```python
from build123d import *

# Parameters (mm, degrees)
BOSS_EXTRUDE1_DEPTH                               = 3.048
BOSS_EXTRUDE2_DEPTH                               = 29.971999999999998
BOSS_EXTRUDE3_DEPTH                               = 3.048
BOSS_EXTRUDE4_DEPTH                               = 3.048
SKETCH13_W                                        = 29.972
SKETCH13_H                                        = 48.7
BOSS_EXTRUDE5_DEPTH                               = 3.048
CSK_FOR_4_FLAT_HEAD_MACHINE_SCREW_100_D           = 2.9464
CSK_FOR_4_FLAT_HEAD_MACHINE_SCREW_100_CSINK_D     = 5.715
CSK_FOR_4_FLAT_HEAD_MACHINE_SCREW_100_CSINK_ANGLE = 100
CUT_EXTRUDE1_DEPTH                                = 1.397
CUT_EXTRUDE1_DEPTH_BACK                           = 1.397
SKETCH15_R                                        = 9.184035329670005
SKETCH15_R_2                                      = 8.124741076595411
SKETCH15_R_3                                      = 8.201451240556812
SKETCH15_R_4                                      = 5.810172256980604
BOSS_EXTRUDE6_DEPTH                               = 3.048
CSK_FOR_4_FLAT_HEAD_MACHINE_SCREW1_AT_2_COUNT     = 2
CSK_FOR_4_FLAT_HEAD_MACHINE_SCREW1_AT_2_PITCH     = 35.474094707842795
CSK_FOR_4_FLAT_HEAD_MACHINE_SCREW1_AT_3_COUNT     = 2
CSK_FOR_4_FLAT_HEAD_MACHINE_SCREW1_AT_3_PITCH     = 43.70753982500484
CSK_FOR_4_FLAT_HEAD_MACHINE_SCREW1_AT_4_COUNT     = 2
CSK_FOR_4_FLAT_HEAD_MACHINE_SCREW1_AT_4_PITCH     = 25.069264350610375
CUT_EXTRUDE2_DEPTH                                = 3.048
FILLET3_R                                         = 3.8099999999999996
FILLET4_R                                         = 1.27
SKETCH21_W                                        = 2.540000000000001
SKETCH21_H                                        = 33.02
CUT_EXTRUDE3_DEPTH                                = 77.47
FILLET5_R                                         = 0.508
FILLET6_R                                         = 0.508
SKETCH22_W                                        = 123.04970813102194
SKETCH22_H                                        = 134.7131875745612
CUT_EXTRUDE4_DEPTH                                = 61.72200000000001


with BuildPart() as part:
    # Sketch2 → Boss-Extrude1 (new body)
    with BuildSketch(Plane.XY):
        Polygon((-47.58059551455695, 48.12489153745831), (-22.21147896413696, 6.554494312375088), (5.701292889255674, 23.58878817682547), (-19.667823661164306, 65.1591854019087), align=None)
        Polygon((-38.85234269167306, 46.0124042215628), (-20.098991648241444, 15.282747135258976), (-3.0269599336282123, 25.701275492720985), (-21.78031097705982, 56.430932579024805), align=None, mode=Mode.SUBTRACT)
    extrude(amount=BOSS_EXTRUDE1_DEPTH)

    # Sketch3 → Boss-Extrude2 (add)
    with BuildSketch(Plane.XY.offset(3.048)):
        Polygon((2.4490708476218597, 21.604058524728963), (-22.920045702798127, 63.17445574981219), (-44.328373472923126, 50.10962118955482), (-18.95925692250314, 8.539223964471608), align=None)
        Polygon((-38.85234269167306, 46.0124042215628), (-20.098991648241444, 15.282747135258976), (-3.0269599336282087, 25.701275492720985), (-21.78031097705982, 56.430932579024805), align=None, mode=Mode.SUBTRACT)
    extrude(amount=BOSS_EXTRUDE2_DEPTH)

    # Sketch4 → Boss-Extrude3 (add)
    with BuildSketch(Plane.XY.offset(33.02)):
        Polygon((-38.85234269167306, 46.0124042215628), (-37.46131723814535, 43.733039051773666), (-20.389285523532113, 54.15156740923567), (-21.78031097705982, 56.430932579024805), align=None)
        Polygon((-29.47566716995725, 30.647575678410885), (-12.403635455344016, 41.0661040358729), (-3.0269599336282087, 25.701275492720985), (-20.098991648241444, 15.282747135258976), align=None)
    extrude(amount=-BOSS_EXTRUDE3_DEPTH)

    # Sketch12 → Boss-Extrude4 (add)
    with BuildSketch(Plane.XY.offset(3.048)):
        Polygon((2.4490708476218597, 21.604058524728963), (5.701292889255674, 23.58878817682547), (8.120429940678708, 25.065112049236276), (-17.248686609741274, 66.6355092743195), (-22.920045702798127, 63.17445574981219), align=None)
    extrude(amount=-BOSS_EXTRUDE4_DEPTH)

    # Sketch13 → Boss-Extrude5 (add)
    with BuildSketch(Plane(origin=(11.391019162328917, 6.95158362794815, 0), x_dir=(0, 0, -1), z_dir=(0.8536015857306615, 0.5209264178731006, 0))):
        with Locations((-18.034000000000002, 41.515472911157566)):
            Rectangle(SKETCH13_W, SKETCH13_H)
    extrude(amount=BOSS_EXTRUDE5_DEPTH)

    # CSK for #4 Flat Head Machine Screw (100)2 (through all)
    with Locations(Plane(origin=(-10.017308607796087, -6.113250932309213, 0), x_dir=(0, 0, 1), z_dir=(-0.8536015857306615, -0.5209264178731007, 0))):
        with Locations((27.397617355, 61.471448289), (7.925915452, 61.471448289), (7.925915452, 21.515515982), (27.397617355, 21.515515982)):
            CounterSinkHole(CSK_FOR_4_FLAT_HEAD_MACHINE_SCREW_100_D / 2, CSK_FOR_4_FLAT_HEAD_MACHINE_SCREW_100_CSINK_D / 2, counter_sink_angle=CSK_FOR_4_FLAT_HEAD_MACHINE_SCREW_100_CSINK_ANGLE)

    # Sketch14 → Cut-Extrude1 (cut, two sides: drawn at the far end of the back side and taken through both)
    with BuildSketch(Plane(origin=(11.607833965104508, 7.083898938087922, 0), x_dir=(0, 0, -1), z_dir=(0.8536015857306615, 0.5209264178731005, 0)).offset(-CUT_EXTRUDE1_DEPTH_BACK)):
        Polygon((-30.697174143874744, 19.61051598216394), (-30.697174143874744, 14.979833054183299), (-24.09806056703731, 14.979833054183299), (-24.09806056703731, 19.610515982163985), (-24.098060567037347, 23.42051598216399), (-27.39761735545604, 25.325515982163957), (-30.697174143874758, 23.420515982163952), align=None)
        Polygon((-27.39761735545604, 57.661448288693826), (-24.098060567037333, 59.56644828869383), (-24.098060567037336, 63.37644828869381), (-24.098060567037336, 70.99644828869384), (-30.69717414387474, 70.99644828869384), (-30.69717414387474, 63.37644828869381), (-30.69717414387474, 59.56644828869381), align=None)
        Polygon((-7.925915451689084, 57.661448288693826), (-4.626358663270381, 59.56644828869382), (-4.626358663270402, 63.37644828869381), (-4.626358663270402, 70.99644828869384), (-11.225472240107786, 70.99644828869384), (-11.225472240107786, 63.376448288693766), (-11.225472240107747, 59.566448288693785), align=None)
        Polygon((-7.925915451689081, 25.325515982163946), (-11.225472240107791, 23.42051598216395), (-11.225472240107791, 19.610515982163946), (-11.225472240107791, 14.979833054183299), (-4.626358663270366, 14.979833054183299), (-4.626358663270366, 19.610515982163953), (-4.6263586632703655, 23.420515982163952), align=None)
    extrude(amount=CUT_EXTRUDE1_DEPTH + CUT_EXTRUDE1_DEPTH_BACK, mode=Mode.SUBTRACT)

    # Sketch15 → Boss-Extrude6 (add)
    with BuildSketch(Plane(origin=(0, 0, 0), x_dir=(-1, 0, 0), z_dir=(0, 0, -1))):
        with Locations((9.758086495919196, 54.36124573948299)):
            Circle(SKETCH15_R)
        with Locations((39.927818301519274, 35.58488100974543)):
            Circle(SKETCH15_R_2)
        with Locations((25.610425726235285, 18.04643091882164)):
            Circle(SKETCH15_R_3)
        with Locations((-3.4576236647063787, 32.70568986323082)):
            Circle(SKETCH15_R_4)
    extrude(amount=-BOSS_EXTRUDE6_DEPTH)

    # Sketch19 → CSK for #4 Flat Head Machine Screw1 (revolve, cut)
    with BuildSketch(Plane(origin=(3.764373982237945, 32.86032278852424, 3.048), x_dir=(0, -1, 0), z_dir=(1, 0, 0))):
        Polygon((0, 0), (-7.5e-16, 3.0480000000000023), (1.4731999999999932, 3.0480000000000023), (1.4731999999999934, 1.59245498611605), (2.857499999999999, -1.73e-15), align=None)
    csk_for_4_flat_head_machine_screw1 = revolve(axis=Axis((3.764373982237945, 32.86032278852424, 9.39799999999999), (0, 0, -1)), mode=Mode.SUBTRACT)

    # CSK for #4 Flat Head Machine Screw1 at 2: CSK for #4 Flat Head Machine Screw1 ×2
    with Locations(*[Vector(-0.8506492202713736, -0.5257336816789507, 0) * (i * CSK_FOR_4_FLAT_HEAD_MACHINE_SCREW1_AT_2_PITCH) for i in range(1, CSK_FOR_4_FLAT_HEAD_MACHINE_SCREW1_AT_2_COUNT)]):
        add(csk_for_4_flat_head_machine_screw1, mode=Mode.SUBTRACT)

    # CSK for #4 Flat Head Machine Screw1 at 3: CSK for #4 Flat Head Machine Screw1 ×2
    with Locations(*[Vector(-0.997755305773639, 0.06696528802709796, 0) * (i * CSK_FOR_4_FLAT_HEAD_MACHINE_SCREW1_AT_3_PITCH) for i in range(1, CSK_FOR_4_FLAT_HEAD_MACHINE_SCREW1_AT_3_COUNT)]):
        add(csk_for_4_flat_head_machine_screw1, mode=Mode.SUBTRACT)

    # CSK for #4 Flat Head Machine Screw1 at 4: CSK for #4 Flat Head Machine Screw1 ×2
    with Locations(*[Vector(-0.5210117203175807, 0.8535495224600124, 0) * (i * CSK_FOR_4_FLAT_HEAD_MACHINE_SCREW1_AT_4_PITCH) for i in range(1, CSK_FOR_4_FLAT_HEAD_MACHINE_SCREW1_AT_4_COUNT)]):
        add(csk_for_4_flat_head_machine_screw1, mode=Mode.SUBTRACT)

    # Sketch20 → Cut-Extrude2 (cut)
    with BuildSketch(Plane(origin=(0, 0, 0), x_dir=(-1, 0, 0), z_dir=(0, 0, -1))):
        with BuildLine():
            Line((14.542293121824187, 62.20075286029573), (11.563953125478477, 57.32037886408755))
            ThreePointArc((11.563953125478477, 57.32037886408755), (6.044784522535942, 56.24291105550805), (7.610320649443919, 50.84186897257834))
            Line((7.610320649443919, 50.84186897257834), (-1.4954062126549716, 35.92102291440944))
            ThreePointArc((-1.4954062126549716, 35.92102291440944), (-7.016596023871767, 34.845052440620755), (-5.448804035753348, 29.442897530407524))
            Line((-5.448804035753348, 29.442897530407524), (-6.484295885760952, 27.746117611303884))
            Line((-6.484295885760952, 27.746117611303884), (-6.762670750549963, 27.28996638176623))
            Line((-6.762670750549963, 27.28996638176623), (-14.061950278269341, 31.74448896114331))
            Line((-14.061950278269341, 31.74448896114331), (8.559037851416688, 68.81174198534737))
            Line((8.559037851416688, 68.81174198534737), (14.542293121824187, 65.16034795406075))
            Line((14.542293121824187, 65.16034795406075), (14.542293121824187, 62.20075286029573))
        make_face()
        Polygon((21.78031097705982, 56.430932579024805), (38.85234269167306, 46.0124042215628), (20.098991648241444, 15.282747135258976), (3.0269599336282123, 25.701275492720985), align=None)
        with BuildLine():
            Line((22.21147896413696, 6.554494312375088), (24.781951964671258, 10.766528400207497))
            ThreePointArc((24.781951964671258, 10.766528400207497), (29.66385906245521, 12.225666721445755), (28.72915433514684, 17.23450177808784))
            Line((28.72915433514684, 17.23450177808784), (38.012718373529104, 32.44675577885475))
            ThreePointArc((38.012718373529104, 32.44675577885475), (43.097277822107074, 33.802481129765034), (41.97793801322115, 38.944252653808825))
            Line((41.97793801322115, 38.944252653808825), (47.58059551455695, 48.12489153745831))
            Line((47.58059551455695, 48.12489153745831), (51.80171473929435, 35.787210781861546))
            Line((51.80171473929435, 35.787210781861546), (47.57680035710003, 5.227667032097241))
            Line((47.57680035710003, 5.227667032097241), (22.21147896413696, 6.554494312375088))
        make_face()
    extrude(amount=-CUT_EXTRUDE2_DEPTH, mode=Mode.SUBTRACT)


with BuildPart() as body_2:
    # of the pieces the cut leaves, the one that is kept (cut_extrude2_keep)
    add(part.part.solids().sort_by_distance((-47.580595515, 48.124891537, 0))[0])

    # Fillet3
    fillet3_edges = [body_2.edges().sort_by_distance(p)[0] for p in [
        (-17.248686609741274, 66.6355092743195, 1.524),
        (-47.58059551455695, 48.12489153745831, 1.524),
        (-22.21147896413696, 6.554494312375088, 1.524),
        (8.120429940678708, 25.065112049236276, 1.524),
    ]]
    fillet(fillet3_edges, radius=FILLET3_R)

    # Fillet4
    fillet4_edges = [body_2.edges().sort_by_distance(p)[0] for p in [
        (1.4954062126549714, 35.92102291440944, 1.524),
        (-24.781951964671258, 10.766528400207495, 1.524),
        (-28.72915433514684, 17.23450177808784, 1.524),
        (-38.0127183735291, 32.44675577885475, 1.524),
        (-41.97793801322115, 38.94425265380882, 1.524),
        (-11.563953125478475, 57.320378864087544, 1.524),
        (-7.610320649443917, 50.84186897257834, 1.524),
    ]]
    fillet(fillet4_edges, radius=FILLET4_R)

    # Sketch21 → Cut-Extrude3 (cut)
    with BuildSketch(Plane(origin=(-8.941948314707059, 14.652474896780824, 0), x_dir=(0.8536015857306616, 0.5209264178731006, 0), z_dir=(0.5209264178731005, -0.8536015857306615, 0))):
        with Locations((2.2216732427396275, 16.51)):
            Rectangle(SKETCH21_W, SKETCH21_H)
    extrude(amount=-CUT_EXTRUDE3_DEPTH, mode=Mode.SUBTRACT)


with BuildPart() as cut_extrude3_piece_1:
    # of the separate pieces the step leaves, piece 1, a body of its own (cut_extrude3_pieces)
    add(body_2.part.solids().sort_by_distance((-12.188709065, 58.344117807, 0))[0])

    # Fillet6
    fillet6_edges = [cut_extrude3_piece_1.edges().sort_by_distance(p)[0] for p in [
        (-7.633709794281099, 43.97704085894782, 3.048),
    ]]
    fillet(fillet6_edges, radius=FILLET6_R)

    # Sketch22 → Cut-Extrude4 (cut)
    with BuildSketch(Plane(origin=(2.067982642978631, 1.2620252919381492, 0), x_dir=(0, 0, -1), z_dir=(0.8536015857306616, 0.5209264178731006, 0))):
        with Locations((-42.687564536567926, 74.45417523171726)):
            Rectangle(SKETCH22_W, SKETCH22_H)
    extrude(amount=CUT_EXTRUDE4_DEPTH, mode=Mode.SUBTRACT)


with BuildPart() as cut_extrude3_piece_2:
    # of the separate pieces the step leaves, piece 2, a body of its own (cut_extrude3_pieces)
    add(body_2.part.solids().sort_by_distance((-42.532157132, 39.852408399, 0))[0])

    # Fillet5
    fillet5_edges = [cut_extrude3_piece_2.edges().sort_by_distance(p)[0] for p in [
        (-31.64381519771313, 29.324422577013216, 3.048),
    ]]
    fillet(fillet5_edges, radius=FILLET5_R)


solid = cut_extrude3_piece_2.part
```
Input: part model. Units: mm. Frame: model coordinates. A direction names the side the tool comes from. Give positions to 0.01 mm unless a question says otherwise; leave off trailing zeros. Write each loop counter-clockwise with the first axis right and the second up, starting at its lowest first coordinate (ties: lowest second). Pieces come first, ordered by that corner, then holes. Notation, with made-up numbers: (62.25, 69) - (85.25, 69) arc R21 cw to (85.25, 102) - close; hole circle Ø7 at (45, 69). An arc over 180 degrees is marked (long way). Write item = value, one per line. Start each with the question number.
1) Pin query (flat end, axial travel): pin 1 (5 mm diameter, centred on x = -35.5, z = 6, fed in from +Y); pin 2 (2.5 mm diameter, centred on x = -39.85, y = 35.79, fed in from -Z); pin 3 (4 mm diameter, centred on x = -32.5, y = 47.5, fed in from -Z); pin 4 (10 mm diameter, centred on x = -42, z = 24, fed in from -Y). Return the tip coordinate at first contact, or that it passes through.
2) Reachability of faces 1 (the face through (-35, 29, 3.048)), 2 (the face through (-34.461, 48.692, 14.776)), 3 (the face through (-20, 26, 29.972)), 4 (the face through (-44.085, 42.398, 1.503)) from +Z, -Z, +X, -X, +Y, -Y: full face, straight path, thin tool, end or side. Return the list, or none.
3) Cut plane A-A (z = 18). Return loops of the section in (x, y), and give its area (3 significant figures).
4) Draft query along Y for faces 5 (the face through (-30, 31, 0)), 6 (the face through (-38.989, 53.368, 16.741)), 7 (the face through (-42.35, 39.08, 1.55)). Return one class per face: pulls with the +Y half, pulls with the -Y half, needs draft (parallel to the pull), parting line crosses it, or undercut.
5) Cut plane B-B (x = -12). Give the number of separate pieces and of enclosed holes in the cut face, and give its area (3 significant figures).
6) Material intervals for L1, parallel to Z at x = -34, y = 52; L2, parallel to Y at x = -31.5, z = 10.5; L3, parallel to Z at x = -41, y = 39.5, sorted ascending. Write a range as [from, to].
Answers follow:
q1.pin_1 = 56.72
q1.pin_2 = through
q1.pin_3 = 29.97
q1.pin_4 = 38.1
q2.face_1 = +Z, -X, -Y
q2.face_2 = -Z, +X
q2.face_3 = -Z, +Y
q2.face_4 = +Z, -Z, -X
q3.outline = (-44.33, 50.11) - (-18.96, 8.54) - (-8.13, 15.15) - (-11.44, 20.57) - (-20.1, 15.28) - (-38.85, 46.01) - (-30.19, 51.3) - (-33.5, 56.72) - close
q3.area = 253 mm^2
q4.face_5 = needs draft
q4.face_6 = pulls with the +Y half
q4.face_7 = undercut
q5.separate_pieces = 1
q5.enclosed_holes = 2
q5.area = 234 mm^2
q6.L1 = [0, 6.59], [9.26, 26.06], [28.73, 33.02]
q6.L2 = [29.09, 33.96], [50.5, 53.44]
q6.L3 = [0, 3.05]
